CAD build for the part. Positions are in the model's coordinates, mm. Face numbers are marked on the shaded views. A direction names the side the tool comes from. Coordinates: 2 decimals unless noted, no trailing zeros. Write each loop counter-clockwise with the first axis right and the second up, starting at its lowest first coordinate (ties: lowest second). Pieces come first, ordered by that corner, then holes. Notation, with made-up numbers: (81, 87.25) -> (104, 87.25) arc R32 ccw to (104, 121.25) -> close; hole circle Ø4 at (56, 40). An arc over 180 degrees is marked (long way). Answer as CSV lines item,"result".
```python
from build123d import *

# Parameters (mm, degrees)
BOSS_EXTRUDE1_DEPTH = 25
CUT_EXTRUDE1_DEPTH  = 22
CHAMFER1_SIZE       = 10
FILLET1_R           = 2
FILLET2_R           = 5
CUT_EXTRUDE4_DEPTH  = 0.5
BOSS_EXTRUDE2_DEPTH = 7
BOSS_EXTRUDE3_DEPTH = 7
BOSS_EXTRUDE4_DEPTH = 7
BOSS_EXTRUDE5_DEPTH = 7
SKETCH10_W          = 3
SKETCH10_H          = 6
CUT_EXTRUDE5_DEPTH  = 123.16586282655703
FILLET3_R           = 3


with BuildPart() as part:
    # Sketch1 → Boss-Extrude1 (new body)
    with BuildSketch(Plane(origin=(0, 0, 0), x_dir=(1, 0, 0), z_dir=(0, 1, 0))):
        Polygon((19, -95), (19, 6.9154344510577115), (-43.296040452526896, 81.15696446475283), (-72.40572929104839, 56.73103529666472), (-18.999999999999996, -6.915434451057793), (-19, -95), align=None)
    extrude(amount=BOSS_EXTRUDE1_DEPTH)

    # Sketch2 → Cut-Extrude1 (cut)
    with BuildSketch(Plane(origin=(0, 25, 0), x_dir=(1, 0, 0), z_dir=(0, 1, 0))):
        Polygon((-68.17923313263185, 56.36126479636737), (-43.66581095282428, 76.93046830633632), (16, 5.823523748259106), (16.00000000000001, -92), (-15.99999999999999, -92), (-15.999999999999996, -5.823523748259207), align=None)
    extrude(amount=-CUT_EXTRUDE1_DEPTH, mode=Mode.SUBTRACT)

    # Chamfer1
    chamfer1_edges = [part.edges().sort_by_distance(p)[0] for p in [
        (-42.089616566315925, 3, -25.26887052405408),
        (-55.92252204272806, 3, -66.64586655135184),
        (-13.83290547641214, 3, -41.376996027297714),
        (16.000000000000007, 3, 43.08823812587045),
        (1.066e-14, 3, 92),
        (-15.999999999999993, 3, 48.9117618741296),
        (-18.999999999999996, 0, 50.957717225528896),
        (-45.7028646455242, 0, -24.90780042280347),
        (-57.85088487178764, 0, -68.94399988070877),
        (-12.148020226263444, 0, -44.036199457905276),
        (19, 0, 44.04228277447115),
        (0, 0, 95),
    ]]
    chamfer(chamfer1_edges, length=CHAMFER1_SIZE)

    # Fillet1
    fillet1_edges = [part.edges().sort_by_distance(p)[0] for p in [
        (19, 17.5, -6.9154344510577115),
        (-68.17923313263185, 19, -56.36126479636737),
        (-43.66581095282428, 19, -76.93046830633632),
        (16.00000000000001, 19, 92),
        (-15.99999999999999, 19, 92),
        (-15.999999999999996, 19, 5.823523748259207),
    ]]
    fillet(fillet1_edges, radius=FILLET1_R)

    # Fillet2
    fillet2_edges = [part.edges().sort_by_distance(p)[0] for p in [
        (-19, 17.5, 95),
        (-18.999999999999996, 17.5, 6.915434451057793),
        (-72.40572929104839, 17.5, -56.73103529666472),
        (-43.296040452526896, 17.5, -81.15696446475283),
        (19, 17.5, 95),
        (16, 19, -5.823523748259106),
    ]]
    fillet(fillet2_edges, radius=FILLET2_R)

    # Sketch9 → Cut-Extrude4 (cut)
    with BuildSketch(Plane.XY.offset(95)):
        Polygon((0.4844994416495535, 15.096060671986343), (0.03578149293160474, 15.096060671986343), (0.03578149293160474, 18.19221451814019), (-1.2655005583504468, 18.19221451814019), (-1.2655005583504468, 18.596060671986343), (0.4844994416495535, 18.596060671986343), align=None)
    extrude(amount=-CUT_EXTRUDE4_DEPTH, mode=Mode.SUBTRACT)

    # Sketch3 → Boss-Extrude2 (add)
    with BuildSketch(Plane(origin=(-14.554844419260807, 0, 12.212964584044096), x_dir=(0.6427876096865288, 0, 0.766044443118987), z_dir=(-0.766044443118987, 0, 0.6427876096865288))):
        Polygon((-68, 15.000000000000004), (-82.00000000000001, 15.000000000000002), (-82.00000000000001, 25), (-68.00000000000001, 25), align=None)
    extrude(amount=BOSS_EXTRUDE2_DEPTH)

    # Sketch4 → Boss-Extrude3 (add)
    with BuildSketch(Plane(origin=(14.554844419260744, 0, -12.212964584044062), x_dir=(-0.6427876096865294, 0, -0.7660444431189866), z_dir=(0.7660444431189866, 0, -0.6427876096865294))):
        Polygon((82.00000000000001, 15.000000000000002), (68.00000000000001, 14.999999999999998), (68.00000000000001, 25), (82.00000000000001, 25), align=None)
    extrude(amount=BOSS_EXTRUDE3_DEPTH)

    # Sketch6 → Boss-Extrude4 (add)
    with BuildSketch(Plane.ZY.offset(18.999999999999996)):
        Polygon((87, 15.000000000000002), (73, 15), (72.99999999999999, 25), (87, 25), align=None)
    extrude(amount=BOSS_EXTRUDE4_DEPTH)

    # Sketch7 → Boss-Extrude5 (add)
    with BuildSketch(Plane(origin=(19, 0, 0), x_dir=(0, 0, -1), z_dir=(1, 0, 0))):
        Polygon((-73, 15.000000000000004), (-87, 15.000000000000002), (-87, 25), (-73, 25), align=None)
    extrude(amount=BOSS_EXTRUDE5_DEPTH)

    # Sketch10 → Cut-Extrude5 (cut, through all)
    with BuildSketch(Plane(origin=(0, 25, 0), x_dir=(1, 0, 0), z_dir=(0, 1, 0))):
        Polygon((-66.99041130416701, 45.61013915017732), (-64.69227797481005, 47.53850197923691), (-60.83555231669091, 42.942235320523), (-63.13368564604784, 41.013872491463395), align=None)
        Polygon((-35.582589136288576, 71.96443114732502), (-33.28445580693161, 73.8927939763846), (-29.427730148812422, 69.29652731767068), (-31.725863478169394, 67.3681644886111), align=None)
        with Locations((-20.499999999999996, -79.99999999999999)):
            Rectangle(SKETCH10_W, SKETCH10_H)
        with Locations((20.5, -80)):
            Rectangle(SKETCH10_W, SKETCH10_H)
    extrude(amount=-CUT_EXTRUDE5_DEPTH, mode=Mode.SUBTRACT)

    # Fillet3
    fillet3_edges = [part.edges().sort_by_distance(p)[0] for p in [
        (-58.26440187794476, 20, -39.878057548047025),
        (-65.97785319418313, 15.000000000000002, -49.07059086547488),
        (19, 20, 87),
        (19, 15.000000000000004, 75),
        (-18.999999999999996, 20, 87),
        (-18.999999999999996, 20, 73),
        (-29.154713039423243, 20, -64.30398671613516),
        (-38.153739575034656, 20, -75.02860891980096),
        (-60.94555742886122, 15.000000000000004, -37.62830091414418),
        (-59.549977097317836, 15.000000000000004, -41.410146434285004),
        (-63.62671297977768, 20, -35.37854428024132),
        (-67.26342841355618, 20, -50.60267975171285),
        (-72.62573951538909, 20, -46.103166483907145),
        (-68.12622624758338, 15.000000000000004, -40.74085538207423),
        (-69.94458396447264, 15.000000000000002, -48.35292311781),
        (26, 20, 87),
        (22.5, 15.000000000000002, 87),
        (19, 15.000000000000002, 85),
        (26, 15.000000000000004, 80),
        (19, 20, 73),
        (22.5, 15.000000000000004, 73),
        (26, 20, 73),
        (-25.999999999999996, 20, 87),
        (-22.499999999999996, 15.000000000000002, 87),
        (-18.999999999999996, 15.000000000000002, 85),
        (-18.999999999999996, 15, 75),
        (-25.999999999999996, 15, 80),
        (-25.999999999999996, 20, 73),
        (-22.499999999999996, 15, 73),
        (-30.440288258796315, 14.999999999999998, -65.83607560237314),
        (-26.47355748850679, 14.999999999999998, -66.553743350038),
        (-23.792401937590338, 20, -68.80349998394087),
        (-35.472584024118206, 15.000000000000002, -77.27836555370381),
        (-28.29191520539604, 15, -74.16581108577375),
        (-36.868164355661605, 15.000000000000002, -73.496520033563),
        (-32.79142847320175, 20, -79.52812218760667),
    ]]
    fillet(fillet3_edges, radius=FILLET3_R - 0.0001)  # a hair under: the kernel refuses the full size


solid = part.part
```
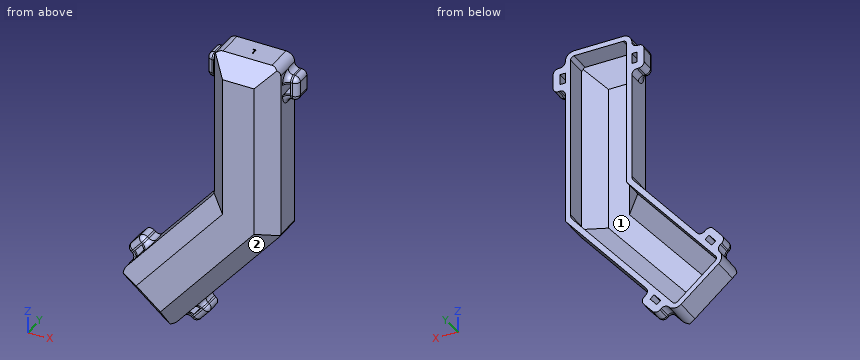
Item 1: 3-axis set-ups, long thin cutter, end or side, ignore diameter. For the marked faces 1 and 2: which of +Z, -Z, +X, -X, +Y, -Y reach the whole face in a straight line?
Answer below:
face 1,"+Y"
face 2,"-Z, +X, -Y"
Item 2: Saw through at A-A on z = 52. Give the cut face in (x, y), and give its area (3 significant figures).
Answer below:
outline,"(-19, 10) -> (-9, 0) -> (9, 0) -> (19, 10) -> (19, 25) -> (16, 25) -> (16, 13) -> (6, 3) -> (-6, 3) -> (-16, 13) -> (-16, 25) -> (-19, 25) -> close"
area,"246 mm2"
Item 3: Saw through at B-B on y = 6.25. Give the cut face in (x, z), and give its area (3 significant figures).
Answer below:
outline,"(-67.12, -56.27) -> (-43.76, -75.87) -> (15.25, -5.55) -> (15.25, 91.25) -> (-15.25, 91.25) -> (-15.25, 5.55) -> close; hole (-58.67, -55.53) -> (-44.5, -67.42) -> (9.25, -3.37) -> (9.25, 85.25) -> (-9.25, 85.25) -> (-9.25, 3.37) -> close"
area,"2,350 mm2"
Item 4: Saw through at C-C on z = -21. Give the cut face in (x, y), and give its area (3 significant figures).
Answer below:
outline,"(-42.42, 10) -> (-29.37, 0) -> (-5.87, 0) -> (7.18, 10) -> (7.18, 25) -> (3.27, 25) -> (3.27, 13) -> (-9.79, 3) -> (-25.45, 3) -> (-38.51, 13) -> (-38.51, 25) -> (-42.42, 25) -> close"
area,"321 mm2"
Item 5: Flat gauge pins, fed straight in: pin 1 (12 mm diameter, centred on y = 12.5, z = 54.5, fed in from +X); pin 2 (0.8 mm diameter, centred on x = -22.5, y = 23, fed in from -Z); pin 3 (1 mm diameter, centred on y = 21, z = -8, fed in from +X). Where does each tip first touch, or does it go through?
Answer below:
pin 1,"stops at x = 19"
pin 2,"stops at z = -56.85"
pin 3,"stops at x = 18.51"
Item 6: Wall check: line 1 (Z direction, x = -9, y = 13.25); line 2 (X direction, y = 23, z = -46.5); line 3 (Z direction, x = -30.5, y = 19.75). Give the ranges that are in metal, low to high. Write a range as from..to.
Answer below:
line 1,"z = -40.28..-35.62, 92..95"
line 2,"x = -71.3..-65.93, -63.82..-59.9, -18.13..-14.22"
line 3,"z = -76.8..-70.57, -68.4..-61.24, -11.46..-6.79"
